```python
from build123d import *

# Parameters (mm, degrees)
BOSS_EXTRU_1_DEPTH      = 8
ESQUISSE2_R             = 7.15
ENL_V_MAT_EXTRU_1_DEPTH = 265.732643435
ESQUISSE3_R             = 30.35
ENL_V_MAT_EXTRU_4_DEPTH = 4
ESQUISSE4_R             = 7.15
ENL_V_MAT_EXTRU_5_DEPTH = 265.521024684


with BuildPart() as part:
    # Esquisse1 → Boss.-Extru.1 (new, symmetric)
    with BuildSketch(Plane(origin=(0, 0, 0), x_dir=(1, 0, 0), z_dir=(0, 1, 0))):
        with BuildLine():
            Line((-232.15, 30.35), (232.15, 30.35))
            ThreePointArc((232.15, 30.35), (262.5, 0), (232.15, -30.35))
            Line((232.15, -30.35), (-232.15, -30.35))
            ThreePointArc((-232.15, -30.35), (-262.5, 0), (-232.15, 30.35))
        make_face()
    extrude(amount=BOSS_EXTRU_1_DEPTH, both=True)

    # Esquisse2 → Enlèv. mat.-Extru.1 (cut, through all)
    with BuildSketch(Plane(origin=(0, 8, 0), x_dir=(1, 0, 0), z_dir=(0, 1, 0))):
        with Locations(Location((232.15, 0, 0), (0, 0, 270))):
            Circle(ESQUISSE2_R)
    extrude(amount=-ENL_V_MAT_EXTRU_1_DEPTH, mode=Mode.SUBTRACT)

    # Esquisse3 → Enlèv. mat.-Extru.4 (cut)
    with BuildSketch(Plane(origin=(0, 8, 0), x_dir=(1, 0, 0), z_dir=(0, 1, 0))):
        with Locations((-232.15, 0)):
            Circle(ESQUISSE3_R)
    enl_v_mat_extru_4 = extrude(amount=-ENL_V_MAT_EXTRU_4_DEPTH, mode=Mode.SUBTRACT)

    # Symétrie4: Enlèv. mat.-Extru.4 across plane
    add(enl_v_mat_extru_4.mirror(Plane.ZX), mode=Mode.SUBTRACT)

    # Esquisse4 → Enlèv. mat.-Extru.5 (cut, through all)
    with BuildSketch(Plane(origin=(0, 4, 0), x_dir=(1, 0, 0), z_dir=(0, 1, 0))):
        with Locations(Location((-232.15, 0, 0), (0, 0, 270))):
            Circle(ESQUISSE4_R)
    extrude(amount=-ENL_V_MAT_EXTRU_5_DEPTH, mode=Mode.SUBTRACT)


solid = part.part
```
Can you work these out from the model? Positions are in its coordinate system, mm. A direction names the side the tool comes from. Give positions to 0.01 mm unless a question says otherwise; leave off trailing zeros. Write each loop counter-clockwise with the first axis right and the second up, starting at its lowest first coordinate (ties: lowest second). Pieces come first, ordered by that corner, then holes. Notation, with made-up numbers: (-23.75, -37) -> (25.25, -37) arc R20 cw to (25.25, -33) -> close; hole circle Ø5 at (-40, 79.5). An arc over 180 degrees is marked (long way). One line per item, written item: value.
Q1. We'd pull the mould along Z, two halves only. Please class faces 1 (the face through (-3, 0, -30.35)), 2 (the face through (-262.493, 0.056, 0.667)), 3 (the face through (-201.807, -6.028, 0.667)): +Z half, -Z half, draft (parallel to the pull), parting line (faces both ways), or undercut.
Results found:
face 1: -Z half
face 2: parting line
face 3: undercut
Q2. For P1, Ø6, axis at y = 3, z = 23, coming from the +X side; P2, Ø4, axis at y = 2.5, z = -1.5, coming from the -X side; P3, Ø6, axis at y = -6, z = -12, coming from the -X side, each with a flat end and sliding along its axis, tell me the tip position at first contact or that it passes through.
Results found:
P1: stops at x = 254.98
P2: stops at x = -262.5
P3: stops at x = -260.89
Q3. Imagine slicing it at A-A on z = 0. Please give me the cut outline in (x, y).
Results found:
outline: (-262.5, -4) -> (-239.3, -4) -> (-239.3, 4) -> (-262.5, 4) -> close; (-225, -4) -> (-201.8, -4) -> (-201.8, -8) -> (225, -8) -> (225, 8) -> (-201.8, 8) -> (-201.8, 4) -> (-225, 4) -> close; (239.3, -8) -> (262.5, -8) -> (262.5, 8) -> (239.3, 8) -> close
Q4. Imagine slicing it at B-B on y = 1. Please give me the cut outline in (x, z), and give its area (3 significant figures).
Results found:
outline: (-232.15, -30.35) -> (232.15, -30.35) arc R30.35 ccw to (232.15, 30.35) -> (-232.15, 30.35) arc R30.35 ccw to start; hole circle Ø14.3 at (-232.15, 0); hole circle Ø14.3 at (232.15, 0)
area: 30,800 mm^2
Q5. Which directions (+Z, -Z, +X, -X, +Y, -Y) give clear straight access to the entire face, cutting with the end or side of a thin tool? Please do faces 4 (the face through (19, 8, 0)), 5 (the face through (-226, -4, 6)), 6 (the face through (-226, 4, 6)).
Results found:
face 4: +Z, -Z, +X, -X, +Y
face 5: -X, -Y
face 6: -X, +Y
Q6. Please list where these lines run through material, in increasing order: line 1 (X direction, y = -2.25, z = 0); line 2 (X direction, y = 5.5, z = -4); line 3 (X direction, y = -4.75, z = 13). Write a range as [from, to].
Results found:
line 1: x = [-262.5, -239.3], [-225, 225], [239.3, 262.5]
line 2: x = [-202.06, 226.22], [238.08, 262.24]
line 3: x = [-204.73, 259.57]
Q7. Imagine slicing it at C-C on z = -19.5. Please give me the cut outline in (x, y).
Results found:
outline: (-255.41, -4) -> (-208.89, -4) -> (-208.89, -8) -> (255.41, -8) -> (255.41, 8) -> (-208.89, 8) -> (-208.89, 4) -> (-255.41, 4) -> close
